Answer from the drawing. Dimensions are ordinates in mm from the lowest x, y and z of the part. A direction names the side the tool comes from. Coordinates: 2 decimals unless noted, no trailing zeros. Write each loop counter-clockwise with the first axis right and the second up, starting at its lowest first coordinate (ties: lowest second). Pieces come first, ordered by that corner, then holes.
(1) The mould has two halves that part along Z. Classify the marked faces 3, 4, 5 and 6: +Z half, -Z half, draft (parallel to the pull), parting line (faces both ways), or undercut.
(2) Section D-D on y = 6.25 is taken. Write down the section's boundary in (x, z), then the cut area to 3 significant figures.
(3) Which of the six approach directions +Z, -Z, +X, -X, +Y, -Y give full straight-line access (tool end or side, diameter ignored) to the marked faces 1 and 2?
(4) Find the intervals of material crossed by probe 1 along Y at (x, z) = (12.7, 4.75) (1 decimal); probe 2 along Y at (x, z) = (12.7, 20) (1 decimal); probe 3 along Z at (x, y) = (17.5, 23.75), in increasing order.
(5) Given pin 1 (5 mm diameter, centred on x = 11.5, z = 12, fed in from +Y) (3 decimals); pin 2 (3 mm diameter, centred on x = 7, z = 21.5, fed in from -Y); pin 3 (3 mm diameter, centred on x = 10, z = 16.5, fed in from +Y); pin 4 (2 mm diameter, centred on y = 2.5, z = 5, fed in from +X), each flat-ended and moving along its own axis, determine where each tip first touches the part or whether it passes through.
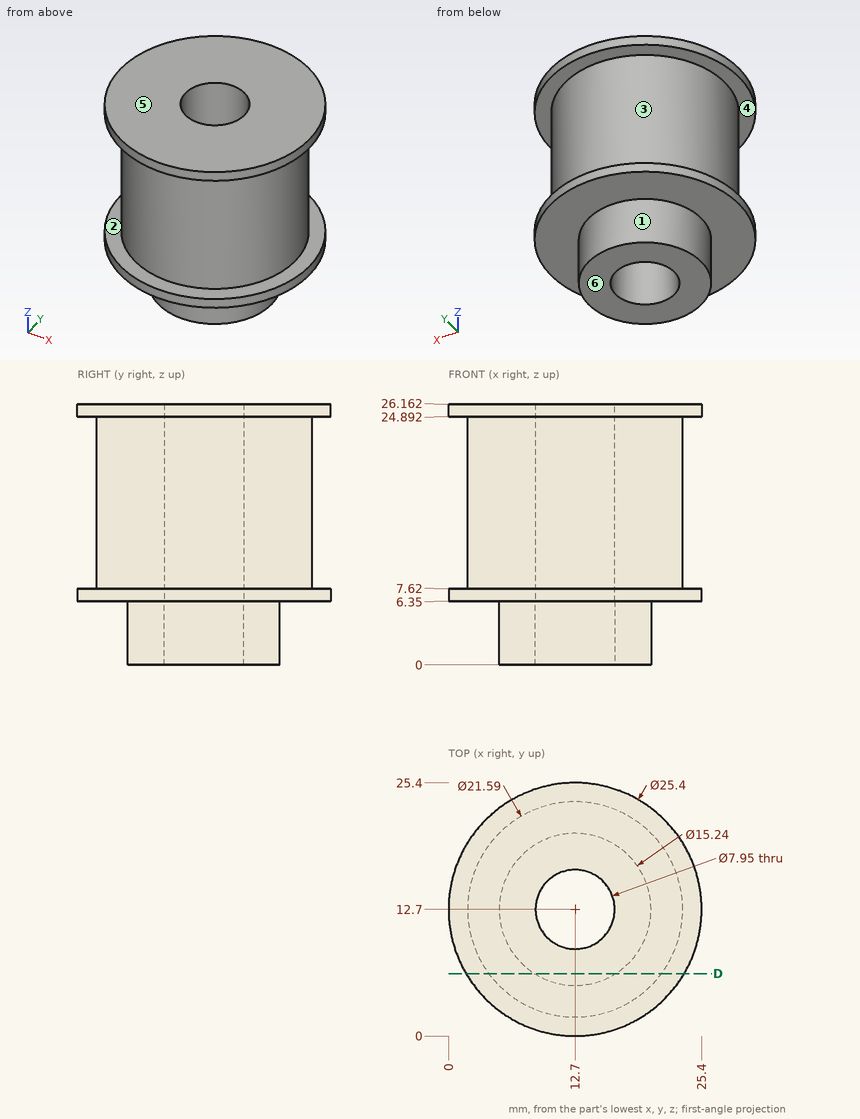
Response:
1. face 3: undercut
1. face 4: undercut
1. face 5: +Z half
1. face 6: -Z half
2. outline: (1.76, 6.35) - (8.64, 6.35) - (8.64, 0) - (16.76, 0) - (16.76, 6.35) - (23.64, 6.35) - (23.64, 7.62) - (21.36, 7.62) - (21.36, 24.89) - (23.64, 24.89) - (23.64, 26.16) - (1.76, 26.16) - (1.76, 24.89) - (4.04, 24.89) - (4.04, 7.62) - (1.76, 7.62) - close
2. area: 406 mm2
3. face 1: -Z
3. face 2: none
4. probe 1: y = 5.1 to 8.7, 16.7 to 20.3
4. probe 2: y = 1.9 to 8.7, 16.7 to 23.5
4. probe 3: z = 6.35 to 7.62, 24.89 to 26.16
5. pin 1: stops at y = 23.495
5. pin 2: stops at y = 2.76
5. pin 3: stops at y = 23.43
5. pin 4: passes through
